Print and shaded views of the part. All mm, measured from the part's lowest x, y and z. A direction names the side the tool comes from. Round coordinates to 2 decimals unless told otherwise and drop trailing zeros. Loops run counter-clockwise (first coordinate to the right, second up) from the corner with the lowest first, then second, coordinate; pieces in that order, holes last. Notation, with made-up numbers: (29.5, 14) - (54.5, 14) arc R26 cw to (54.5, 46) - close; hole circle Ø7 at (-39, 19). An arc over 180 degrees is marked (long way). Use one line per item in the form item = value.
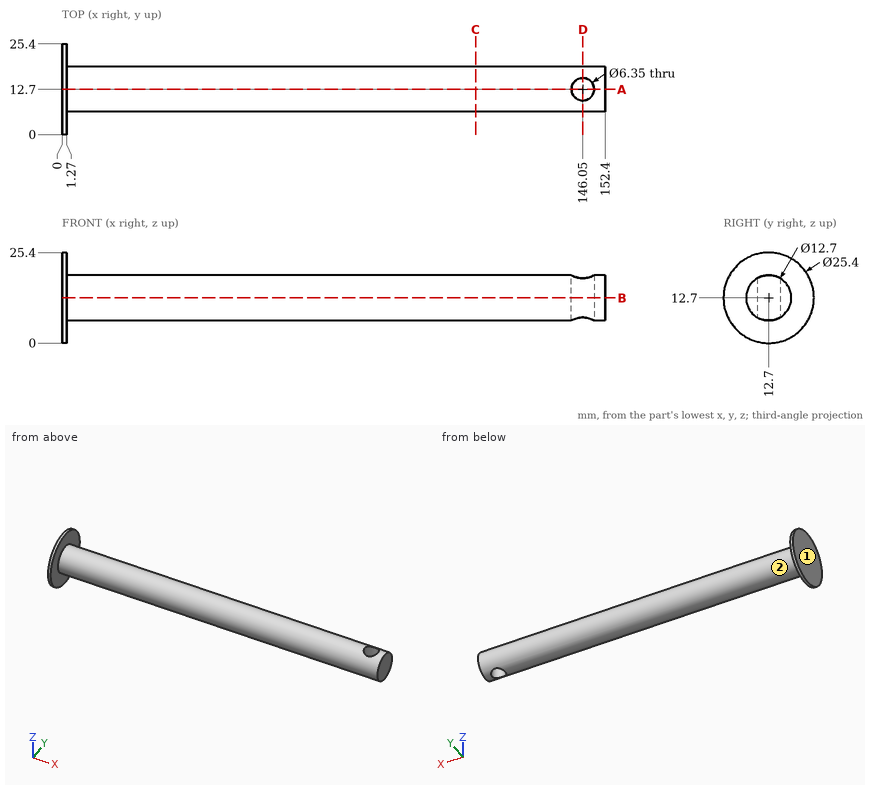
1. Flat gauge pins, fed straight in: pin 1 (2 mm diameter, centred on x = 70, z = 15, fed in from -Y); pin 2 (6 mm diameter, centred on x = 118.5, z = 5.5, fed in from -Y); pin 3 (8 mm diameter, centred on x = 57, y = 22, fed in from +Z). Where does each tip first touch, or does it go through?
Geometry check:
pin_1 = 6.48
pin_2 = 7.94
pin_3 = 16.2
2. Tool access for the marked faces 1 and 2: list every direction of +Z, -Z, +X, -X, +Y, -Y with a clear straight run to the whole face (end or side of a thin tool).
Geometry check:
face_1 = +Z, -Z, -X, +Y, -Y
face_2 = +X
3. Cut at D-D, the plane x = 146.05. Give the cut face in (y, z) (3 decimals).
Geometry check:
outline = (9.525, 7.201) - (9.525, 18.199) arc R6.35 ccw to start; (15.875, 7.201) arc R6.35 ccw to (15.875, 18.199) - close
4. Wall check: probe 1 along X at (y, z) = (12.7, 9.5) (3 decimals); probe 2 along Y at (x, z) = (146.05, 12.5) (3 decimals); probe 3 along X at (y, z) = (2.5, 10.5). Give the ranges that are in metal, low to high.
Geometry check:
probe_1 = 0 to 142.875, 149.225 to 152.4
probe_2 = 6.353 to 9.525, 15.875 to 19.047
probe_3 = 0 to 1.27
5. Cut at B-B, the plane z = 12.7. Give the cut face in (x, y) (3 decimals), plus the area to 3 significant figures.
Geometry check:
outline = (0, 0) - (1.27, 0) - (1.27, 6.35) - (152.4, 6.35) - (152.4, 19.05) - (1.27, 19.05) - (1.27, 25.4) - (0, 25.4) - close; hole circle Ø6.35 at (146.05, 12.7)
area = 1,920 mm^2
6. Cut at C-C, the plane x = 116. Give the cut face in (y, z), plus the area to 3 significant figures.
Geometry check:
outline = circle Ø12.7 at (12.7, 12.7)
area = 127 mm^2
7. Cut at A-A, the plane y = 12.7. Give the cut face in (x, z) (3 decimals).
Geometry check:
outline = (0, 0) - (1.27, 0) - (1.27, 6.35) - (142.875, 6.35) - (142.875, 19.05) - (1.27, 19.05) - (1.27, 25.4) - (0, 25.4) - close; (149.225, 6.35) - (152.4, 6.35) - (152.4, 19.05) - (149.225, 19.05) - close
